```python
from build123d import *

# Parameters (mm, degrees)
F2_DEPTH = 23.25
F3_DEPTH = 41
F4_DEPTH = 72.5
F5_DEPTH = 74
F6_DEPTH = 157
F7_D     = 6.5
F7_DEPTH = 20.001
F8_D     = 6.5


with BuildPart() as f2:
    # F0 (on Front) → F2 (new body)
    with BuildSketch(Plane.XZ):
        Polygon((-9.25, 31.9843477787), (-20, 23.0156522213), (-11.7989976847, 23.0156522213), align=None)
        with BuildLine():
            Line((-11.7989976847, 23.0156522213), (-20, 23.0156522213))
            Line((-20, 23.0156522213), (-20, -23.0156522213))
            Line((-20, -23.0156522213), (-19, -23.0156522213))
            ThreePointArc((-19, -23.0156522213), (0, -4.0156522213), (19, -23.0156522213))
            Line((19, -23.0156522213), (20, -23.0156522213))
            Line((20, -23.0156522213), (20, 23.0156522213))
            Line((20, 23.0156522213), (11.7989976847, 23.0156522213))
            Line((11.7989976847, 23.0156522213), (14.65, 12.9843477787))
            ThreePointArc((14.65, 12.9843477787), (0, -1.7589444033), (-14.65, 12.9843477787))
            Line((-14.65, 12.9843477787), (-11.7989976847, 23.0156522213))
        make_face()
        Polygon((-9.25, 31.9843477787), (-11.7989976847, 23.0156522213), (11.7989976847, 23.0156522213), (9.25, 31.9843477787), align=None)
        with BuildLine():
            Line((-19, -23.0156522213), (-20, -23.0156522213))
            ThreePointArc((-20, -23.0156522213), (0, -43.0156522213), (20, -23.0156522213))
            Line((20, -23.0156522213), (19, -23.0156522213))
            ThreePointArc((19, -23.0156522213), (0, -42.0156522213), (-19, -23.0156522213))
        make_face()
        Polygon((9.25, 31.9843477787), (11.7989976847, 23.0156522213), (20, 23.0156522213), align=None)
        with BuildLine():
            Line((-10, 12.9843477787), (-14.65, 12.9843477787))
            ThreePointArc((-14.65, 12.9843477787), (0, -1.7589444033), (14.65, 12.9843477787))
            Line((14.65, 12.9843477787), (10, 12.9843477787))
            ThreePointArc((10, 12.9843477787), (9.5475471091, 10.0104035628), (8.2311311601, 7.3055732784))
            ThreePointArc((8.2311311601, 7.3055732784), (7.1401280605, 5.8442197181), (5.6787745002, 4.7532166185))
            ThreePointArc((5.6787745002, 4.7532166185), (0, 2.9843477787), (-5.6787745002, 4.7532166185))
            ThreePointArc((-5.6787745002, 4.7532166185), (-7.1401280605, 5.8442197181), (-8.2311311601, 7.3055732784))
            ThreePointArc((-8.2311311601, 7.3055732784), (-9.5475471091, 10.0104035628), (-10, 12.9843477787))
        make_face()
        with BuildLine():
            Line((11.7989976847, 23.0156522213), (-11.7989976847, 23.0156522213))
            Line((-11.7989976847, 23.0156522213), (-14.65, 12.9843477787))
            Line((-14.65, 12.9843477787), (-10, 12.9843477787))
            ThreePointArc((-10, 12.9843477787), (-9.5475471091, 15.9582919946), (-8.2311311601, 18.6631222789))
            ThreePointArc((-8.2311311601, 18.6631222789), (-7.1401280605, 20.1244758392), (-5.6787745002, 21.2154789388))
            ThreePointArc((-5.6787745002, 21.2154789388), (0, 22.9843477787), (5.6787745002, 21.2154789388))
            ThreePointArc((5.6787745002, 21.2154789388), (7.1401280605, 20.1244758392), (8.2311311601, 18.6631222789))
            ThreePointArc((8.2311311601, 18.6631222789), (9.5475471091, 15.9582919946), (10, 12.9843477787))
            Line((10, 12.9843477787), (14.65, 12.9843477787))
            Line((14.65, 12.9843477787), (11.7989976847, 23.0156522213))
        make_face()
        with BuildLine():
            ThreePointArc((5.6787745002, 21.2154789388), (0, 22.9843477787), (-5.6787745002, 21.2154789388))
            ThreePointArc((-5.6787745002, 21.2154789388), (-4.2124207393, 21.7891297759), (-2.65, 21.9843477787))
            Line((-2.65, 21.9843477787), (2.65, 21.9843477787))
            ThreePointArc((2.65, 21.9843477787), (4.2124207393, 21.7891297759), (5.6787745002, 21.2154789388))
        make_face()
        with BuildLine():
            ThreePointArc((-8.2311311601, 18.6631222789), (-9.5475471091, 15.9582919946), (-10, 12.9843477787))
            Line((-10, 12.9843477787), (-9, 12.9843477787))
            Line((-9, 12.9843477787), (-9, 15.6343477787))
            ThreePointArc((-9, 15.6343477787), (-8.8047819972, 17.1967685179), (-8.2311311601, 18.6631222789))
        make_face()
        with BuildLine():
            Line((-9, 12.9843477787), (-10, 12.9843477787))
            ThreePointArc((-10, 12.9843477787), (-9.5475471091, 10.0104035628), (-8.2311311601, 7.3055732784))
            ThreePointArc((-8.2311311601, 7.3055732784), (-8.8047819972, 8.7719270394), (-9, 10.3343477787))
            Line((-9, 10.3343477787), (-9, 12.9843477787))
        make_face()
        with BuildLine():
            ThreePointArc((8.2311311601, 7.3055732784), (9.5475471091, 10.0104035628), (10, 12.9843477787))
            Line((10, 12.9843477787), (9, 12.9843477787))
            Line((9, 12.9843477787), (9, 10.3343477787))
            ThreePointArc((9, 10.3343477787), (8.8047819972, 8.7719270394), (8.2311311601, 7.3055732784))
        make_face()
        with BuildLine():
            Line((9, 12.9843477787), (10, 12.9843477787))
            ThreePointArc((10, 12.9843477787), (9.5475471091, 15.9582919946), (8.2311311601, 18.6631222789))
            ThreePointArc((8.2311311601, 18.6631222789), (8.8047819972, 17.1967685179), (9, 15.6343477787))
            Line((9, 15.6343477787), (9, 12.9843477787))
        make_face()
        with BuildLine():
            ThreePointArc((-2.65, 3.9843477787), (-4.2124207393, 4.1795657814), (-5.6787745002, 4.7532166185))
            ThreePointArc((-5.6787745002, 4.7532166185), (0, 2.9843477787), (5.6787745002, 4.7532166185))
            ThreePointArc((5.6787745002, 4.7532166185), (4.2124207393, 4.1795657814), (2.65, 3.9843477787))
            Line((2.65, 3.9843477787), (-2.65, 3.9843477787))
        make_face()
        with BuildLine():
            ThreePointArc((19, -23.0156522213), (0, -4.0156522213), (-19, -23.0156522213))
            Line((-19, -23.0156522213), (-6.375, -23.0156522213))
            ThreePointArc((-6.375, -23.0156522213), (0, -16.6406522213), (6.375, -23.0156522213))
            Line((6.375, -23.0156522213), (19, -23.0156522213))
        make_face()
        with BuildLine():
            ThreePointArc((6.375, -23.0156522213), (0, -16.6406522213), (-6.375, -23.0156522213))
            Line((-6.375, -23.0156522213), (6.375, -23.0156522213))
        make_face()
        with BuildLine():
            Line((6.375, -23.0156522213), (-6.375, -23.0156522213))
            ThreePointArc((-6.375, -23.0156522213), (0, -29.3906522213), (6.375, -23.0156522213))
        make_face()
        with BuildLine():
            Line((-6.375, -23.0156522213), (-19, -23.0156522213))
            ThreePointArc((-19, -23.0156522213), (0, -42.0156522213), (19, -23.0156522213))
            Line((19, -23.0156522213), (6.375, -23.0156522213))
            ThreePointArc((6.375, -23.0156522213), (0, -29.3906522213), (-6.375, -23.0156522213))
        make_face()
    extrude(amount=F2_DEPTH)

    # F0 (on Front) → F3 (join)
    with BuildSketch(Plane.XZ):
        with BuildLine():
            ThreePointArc((-5.6787745002, 21.2154789388), (-7.0710678119, 20.0554155905), (-8.2311311601, 18.6631222789))
            ThreePointArc((-8.2311311601, 18.6631222789), (-8.8047819972, 17.1967685179), (-9, 15.6343477787))
            Line((-9, 15.6343477787), (-9, 12.9843477787))
            Line((-9, 12.9843477787), (0, 12.9843477787))
            Line((0, 12.9843477787), (9, 12.9843477787))
            Line((9, 12.9843477787), (9, 15.6343477787))
            ThreePointArc((9, 15.6343477787), (8.8047819972, 17.1967685179), (8.2311311601, 18.6631222789))
            ThreePointArc((8.2311311601, 18.6631222789), (7.0710678119, 20.0554155905), (5.6787745002, 21.2154789388))
            ThreePointArc((5.6787745002, 21.2154789388), (4.2124207393, 21.7891297759), (2.65, 21.9843477787))
            Line((2.65, 21.9843477787), (-2.65, 21.9843477787))
            ThreePointArc((-2.65, 21.9843477787), (-4.2124207393, 21.7891297759), (-5.6787745002, 21.2154789388))
        make_face()
        with BuildLine():
            ThreePointArc((-9, 10.3343477787), (-8.8047819972, 8.7719270394), (-8.2311311601, 7.3055732784))
            ThreePointArc((-8.2311311601, 7.3055732784), (-7.0710678119, 5.9132799668), (-5.6787745002, 4.7532166185))
            ThreePointArc((-5.6787745002, 4.7532166185), (-4.2124207393, 4.1795657814), (-2.65, 3.9843477787))
            Line((-2.65, 3.9843477787), (2.65, 3.9843477787))
            ThreePointArc((2.65, 3.9843477787), (4.2124207393, 4.1795657814), (5.6787745002, 4.7532166185))
            ThreePointArc((5.6787745002, 4.7532166185), (7.0710678119, 5.9132799668), (8.2311311601, 7.3055732784))
            ThreePointArc((8.2311311601, 7.3055732784), (8.8047819972, 8.7719270394), (9, 10.3343477787))
            Line((9, 10.3343477787), (9, 12.9843477787))
            Line((9, 12.9843477787), (0, 12.9843477787))
            Line((0, 12.9843477787), (-9, 12.9843477787))
            Line((-9, 12.9843477787), (-9, 10.3343477787))
        make_face()
    extrude(amount=F3_DEPTH)

    # F0 (on Front) → F4 (join)
    with BuildSketch(Plane.XZ):
        with BuildLine():
            ThreePointArc((19, -23.0156522213), (0, -4.0156522213), (-19, -23.0156522213))
            Line((-19, -23.0156522213), (-6.375, -23.0156522213))
            ThreePointArc((-6.375, -23.0156522213), (0, -16.6406522213), (6.375, -23.0156522213))
            Line((6.375, -23.0156522213), (19, -23.0156522213))
        make_face()
        with BuildLine():
            Line((-6.375, -23.0156522213), (-19, -23.0156522213))
            ThreePointArc((-19, -23.0156522213), (0, -42.0156522213), (19, -23.0156522213))
            Line((19, -23.0156522213), (6.375, -23.0156522213))
            ThreePointArc((6.375, -23.0156522213), (0, -29.3906522213), (-6.375, -23.0156522213))
        make_face()
    extrude(amount=-F4_DEPTH)

    # F0 (on Front) → F5 (join)
    with BuildSketch(Plane.XZ):
        with BuildLine():
            ThreePointArc((6.375, -23.0156522213), (0, -16.6406522213), (-6.375, -23.0156522213))
            Line((-6.375, -23.0156522213), (6.375, -23.0156522213))
        make_face()
        with BuildLine():
            Line((6.375, -23.0156522213), (-6.375, -23.0156522213))
            ThreePointArc((-6.375, -23.0156522213), (0, -29.3906522213), (6.375, -23.0156522213))
        make_face()
    extrude(amount=-F5_DEPTH)

    # F0 (on Front) → F6 (join)
    with BuildSketch(Plane.XZ):
        Polygon((-9.25, 31.9843477787), (-11.7989976847, 23.0156522213), (11.7989976847, 23.0156522213), (9.25, 31.9843477787), align=None)
        with BuildLine():
            Line((11.7989976847, 23.0156522213), (-11.7989976847, 23.0156522213))
            Line((-11.7989976847, 23.0156522213), (-14.65, 12.9843477787))
            Line((-14.65, 12.9843477787), (-10, 12.9843477787))
            ThreePointArc((-10, 12.9843477787), (-9.5475471091, 15.9582919946), (-8.2311311601, 18.6631222789))
            ThreePointArc((-8.2311311601, 18.6631222789), (-7.1401280605, 20.1244758392), (-5.6787745002, 21.2154789388))
            ThreePointArc((-5.6787745002, 21.2154789388), (0, 22.9843477787), (5.6787745002, 21.2154789388))
            ThreePointArc((5.6787745002, 21.2154789388), (7.1401280605, 20.1244758392), (8.2311311601, 18.6631222789))
            ThreePointArc((8.2311311601, 18.6631222789), (9.5475471091, 15.9582919946), (10, 12.9843477787))
            Line((10, 12.9843477787), (14.65, 12.9843477787))
            Line((14.65, 12.9843477787), (11.7989976847, 23.0156522213))
        make_face()
        with BuildLine():
            Line((-10, 12.9843477787), (-14.65, 12.9843477787))
            ThreePointArc((-14.65, 12.9843477787), (0, -1.7589444033), (14.65, 12.9843477787))
            Line((14.65, 12.9843477787), (10, 12.9843477787))
            ThreePointArc((10, 12.9843477787), (9.5475471091, 10.0104035628), (8.2311311601, 7.3055732784))
            ThreePointArc((8.2311311601, 7.3055732784), (7.1401280605, 5.8442197181), (5.6787745002, 4.7532166185))
            ThreePointArc((5.6787745002, 4.7532166185), (0, 2.9843477787), (-5.6787745002, 4.7532166185))
            ThreePointArc((-5.6787745002, 4.7532166185), (-7.1401280605, 5.8442197181), (-8.2311311601, 7.3055732784))
            ThreePointArc((-8.2311311601, 7.3055732784), (-9.5475471091, 10.0104035628), (-10, 12.9843477787))
        make_face()
    extrude(amount=-F6_DEPTH)

    # F7 (through all, one way)
    with BuildSketch(Plane.YZ):
        with Locations((-33, 13.1192486733)):
            Circle(F7_D / 2)
    extrude(amount=-F7_DEPTH, mode=Mode.SUBTRACT)

    # F8 (through all)
    with Locations(Plane(origin=(0, 0, 0), x_dir=(0, 1, 0), z_dir=(-1, 0, 0))):
        with Locations((-33, -13.1192486733)):
            Hole(F8_D / 2)


solid = f2.part
```
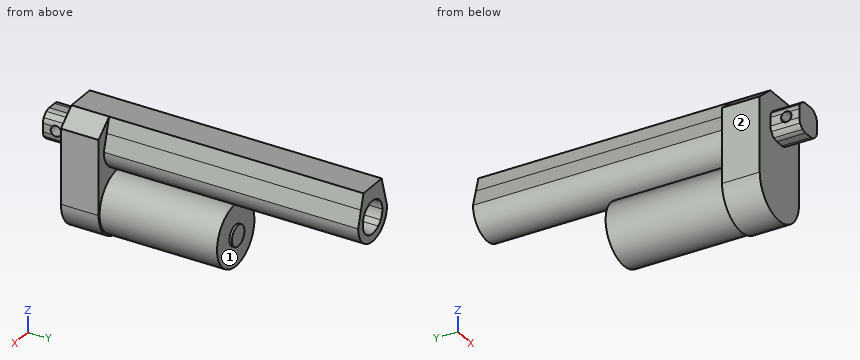
The model under review builds one solid part; all positions refer to its coordinate system, in mm. Face numbers are marked on the shaded views. A direction names the side the tool comes from. Give positions to 0.01 mm unless a question says otherwise; leave off trailing zeros. Loops run counter-clockwise (first coordinate to the right, second up) from the corner with the lowest first, then second, coordinate; pieces in that order, holes last. Notation, with made-up numbers: (-26.75, 71) - (-8.75, 71) arc R17 cw to (-8.75, 89) - close; hole circle Ø3 at (40.5, -17.5). An arc over 180 degrees is marked (long way). Answer as a JSON object with one key per item and string values.
Q1. Insertion check: pin 1 (1.6 mm diameter, centred on y = -38, z = 12, fed in from +X); pin 2 (4 mm diameter, centred on y = -28, z = 13, fed in from -X); pin 3 (1.6 mm diameter, centred on x = 1, y = -35, fed in from -Z); pin 4 (6 mm diameter, centred on y = -33, z = 13.12, fed in from -X). Each pin has a flat end and moves straight along its axis. Give the tip position at first contact, or say it passes through.
Worked out:
{"pin 1": "stops at x = 9", "pin 2": "stops at x = -9", "pin 3": "stops at z = 3.98", "pin 4": "passes through"}
Q2. Add section C-C on y = 141.5. State the section outline as (x, z) points, plus the area to 3 significant figures.
Worked out:
{"outline": "(-14.65, 12.98) arc R14.65 ccw (long way) to (14.65, 12.98) - (9.25, 31.98) - (-9.25, 31.98) - close; hole (-8.23, 7.31) arc R6.35 ccw to (-5.68, 4.75) arc R10 ccw to (5.68, 4.75) arc R6.35 ccw to (8.23, 7.31) arc R10 ccw to (8.23, 18.66) arc R6.35 ccw to (5.68, 21.22) arc R10 ccw to (-5.68, 21.22) arc R6.35 ccw to (-8.23, 18.66) arc R10 ccw to start", "area": "479 mm^2"}
Q3. To check wall thickness, follow line 1 along Y through (x, z) = (-10, 6); line 2 along Z through (x, y) = (2, -33); line 3 along Z through (x, y) = (3.5, 34). State the ranges of each line that lie inside material, in increasing order.
Worked out:
{"line 1": "y = -23.25 to 157", "line 2": "z = 3.98 to 9.87, 16.37 to 21.98", "line 3": "z = -41.69 to -4.34, -1.33 to 3.62, 22.35 to 31.98"}
Q4. For the marked faces 1 and 2, list the 3-axis set-ups (+Z, -Z, +X, -X, +Y, -Y) from which the entire face can be reached by the end or side of a thin tool; tool diameter is ignored.
Worked out:
{"face 1": "+Y", "face 2": "+Z, -Z, -X, +Y, -Y"}
Q5. Add section B-B on y = -7. State the section outline as (x, z) points, plus the area to 3 significant figures.
Worked out:
{"outline": "(-20, -23.02) arc R20 ccw to (20, -23.02) - (20, 23.02) - (9.25, 31.98) - (-9.25, 31.98) - (-20, 23.02) - close; hole (-8.23, 7.31) arc R6.35 ccw to (-5.68, 4.75) arc R10 cw to start; hole (-8.23, 18.66) arc R10 cw to (-5.68, 21.22) arc R6.35 ccw to start; hole (5.68, 4.75) arc R6.35 ccw to (8.23, 7.31) arc R10 cw to start; hole (5.68, 21.22) arc R10 cw to (8.23, 18.66) arc R6.35 ccw to start", "area": "2,730 mm^2"}
Q6. Add section A-A on y = 20. State the section outline as (x, z) points, plus the area to 3 significant figures.
Worked out:
{"outline": "circle Ø38 at (0, -23.02); (-14.65, 12.98) arc R14.65 ccw (long way) to (14.65, 12.98) - (9.25, 31.98) - (-9.25, 31.98) - close; hole (-8.23, 7.31) arc R6.35 ccw to (-5.68, 4.75) arc R10 ccw to (5.68, 4.75) arc R6.35 ccw to (8.23, 7.31) arc R10 ccw to (8.23, 18.66) arc R6.35 ccw to (5.68, 21.22) arc R10 ccw to (-5.68, 21.22) arc R6.35 ccw to (-8.23, 18.66) arc R10 ccw to start", "area": "1,610 mm^2"}
Q7. Add section D-D on z = -13. State the section outline as (x, y) points.
Worked out:
{"outline": "(-20, -23.25) - (20, -23.25) - (20, 0) - (16.15, 0) - (16.15, 72.5) - (-16.15, 72.5) - (-16.15, 0) - (-20, 0) - close"}
